Read the model definition and answer for the solid it produces. Units are mm, in the model's axes. Give positions to 0.01 mm unless a question says otherwise; leave off trailing zeros. Order: outer loops, then holes, each group sorted by start corner. A loop starts at its lowest first (then second) coordinate and runs counter-clockwise, first axis right, second up. Notation, with made-up numbers: (24.5, 35.5) - (76.5, 35.5) arc R11 cw to (76.5, 52.5) - close; hole circle Ø2 at (43, 14.5). An arc over 180 degrees is marked (long way). Write each question's results on one line, items separated by ' | '. Start each with the question number.
Q1. A flat-ended cylindrical pin translates along its axis: P1, Ø1, axis at y = -4, z = 2.5, coming from the -X side. Find the tip coordinate at first contact, or state that the pin passes through.
Q2. Find section A-A on x = 0. Give the vertices of the cut face in (y, z) (3 decimals).
Q3. For a pull along Y with two mould halves and no side action, classify faces 1 (the face through (0, -15, 3)), 2 (the face through (-0.69, 3.1, 3.45)), 3 (the face through (0, -7, 0)), 4 (the face through (-0.079, 4.174, 3.451)) as +Y half, -Y half, draft (parallel to the pull), parting line (faces both ways), or undercut.
Q4. Find the intervals of material crossed by line 1 along Y through (x, z) = (0, 2.5) (3 decimals); line 2 along X through (y, z) = (1.25, 6.25); line 3 along X through (y, z) = (1, 3.75), in increasing order. Write a range as from..to.
Q5. Find section D-D on y = -5. Give the vertices of the cut face in (x, z), and give its area (3 significant figures).
Q6. Find section B-B on y = 0. Give the vertices of the cut face in (x, z) (3 decimals), and give its area (3 significant figures).
Autodesk Inventor part; units mm, degrees
ref_plane "YZ Plane" through (0, 0, 0) normal (1, 0, 0) x (0, 1, 0)
ref_plane "XZ Plane" through (0, 0, 0) normal (0, 1, 0) x (-1, 0, 0)
ref_plane "XY Plane" through (0, 0, 0) normal (0, 0, 1) x (1, 0, 0)
sketch "Boceto1" plane through (0, 0, 0) normal (0, 0, 1) x (1, 0, 0)
  circle A0 centre (0, 0) radius 3.175
  arc A1 (4.0815, 0.8787) -> (-4.0815, 0.8787) centre (0, 0) ccw
  line L0 (0, 0) -> (0, -15) construction
  line L1 (0, -15) -> (7.5, -15) construction
  line L2 (0, -15) -> (-7.5, -15) construction
  line L3 (-7.5, -15) -> (-4.0815, 0.8787)
  line L4 (7.5, -15) -> (4.0815, 0.8787)
  line L5 (7.5, -15) -> (-7.5, -15)
  dimension "d0" = 6.35
  dimension "d1" = 1
  dimension "d2" = 15
  dimension "d3" = 7.5
  dimension "d4" = 7.5
extrude "Extrusión1" add sketch "Boceto1" along normal blind 7
properties part number "base"
Working result:
1) P1: x = -5.24
2) outline: (-15, 0) - (-3.175, 0) - (-3.175, 7) - (-15, 7) - close; (3.175, 0) - (4.175, 0) - (4.175, 7) - (3.175, 7) - close
3) face 1: -Y half | face 2: undercut | face 3: draft | face 4: +Y half
4) line 1: -15..-3.175, 3.175..4.175 | line 2: -3.98..-2.92, 2.92..3.98 | line 3: -4.05..-3.01, 3.01..4.05
5) outline: (-5.35, 0) - (5.35, 0) - (5.35, 7) - (-5.35, 7) - close | area: 74.9 mm²
6) outline: (-4.271, 0) - (-3.175, 0) - (-3.175, 7) - (-4.271, 7) - close; (3.175, 0) - (4.271, 0) - (4.271, 7) - (3.175, 7) - close | area: 15.3 mm²
